Part model, mm, in its own coordinate system. A direction names the side the tool comes from. Give positions to 0.01 mm unless a question says otherwise; leave off trailing zeros. Write each loop counter-clockwise with the first axis right and the second up, starting at its lowest first coordinate (ties: lowest second). Pieces come first, ordered by that corner, then holes.
```python
from build123d import *

# Parameters (mm, degrees)
SKETCH1_R           = 1.4375
BOSS_EXTRUDE1_DEPTH = 5.999988
FILLET3_R           = 7.62
CUT_EXTRUDE2_DEPTH  = 91.763371988
FILLET5_R           = 5.5


with BuildPart() as part:
    # Sketch1 → Boss-Extrude1 (new body)
    # profile 1 of 2: a face of its own
    with BuildSketch(Plane.XY):
        with BuildLine():
            Line((-12.524548321, 23.175850862), (-8.858779162, 0))
            Line((-8.858779162, 0), (79.974319043, 0))
            Line((79.974319043, 0), (82.794220418, 17.828076701))
            ThreePointArc((82.794220418, 17.828076701), (80.81199482, 25.527902595), (73.838835056, 29.347795267))
            Line((73.838835056, 29.347795267), (-2.145190776, 36.382122067))
            ThreePointArc((-2.145190776, 36.382122067), (4.322784828, 33.16197662), (6.932987084, 26.424700516))
            ThreePointArc((6.932987084, 26.424700516), (6.181465859, 22.621328283), (4.039859015, 19.389619041))
            ThreePointArc((4.039859015, 19.389619041), (3.875471285, 19.227345924), (3.707379331, 19.06891302))
            ThreePointArc((3.707379331, 19.06891302), (-5.519878365, 16.730194284), (-12.524548321, 23.175850862))
        make_face()
        with Locations((72.917012916, 19.390373716)):
            Circle(SKETCH1_R, mode=Mode.SUBTRACT)
    # profile 2 of 2: a face of its own
    with BuildSketch(Plane.XY):
        with BuildLine():
            ThreePointArc((-2.145190776, 36.382122067), (-10.929328098, 32.604020866), (-12.524548321, 23.175850862))
            ThreePointArc((-12.524548321, 23.175850862), (-5.519878365, 16.730194284), (3.707379331, 19.06891302))
            ThreePointArc((3.707379331, 19.06891302), (3.875471285, 19.227345924), (4.039859015, 19.389619041))
            ThreePointArc((4.039859015, 19.389619041), (6.181465859, 22.621328283), (6.932987084, 26.424700516))
            ThreePointArc((6.932987084, 26.424700516), (4.322784828, 33.16197662), (-2.145190776, 36.382122067))
        make_face()
        with Locations((-3.067012916, 26.424700516)):
            Circle(SKETCH1_R, mode=Mode.SUBTRACT)
    extrude(amount=BOSS_EXTRUDE1_DEPTH)

    # Fillet3
    fillet3_edges = [part.edges().sort_by_distance(p)[0] for p in [
        (79.974319043, 0, 2.999994),
        (-8.858779162, 0, 2.999994),
    ]]
    fillet(fillet3_edges, radius=FILLET3_R)

    # Sketch3 → Cut-Extrude2 (cut, through all)
    with BuildSketch(Plane.XY.offset(5.999988)):
        Polygon((5.750849923, 35.651135125), (8.226420239, 20), (62.889119642, 20), (64.504363049, 30.211946987), align=None)
    extrude(amount=-CUT_EXTRUDE2_DEPTH, mode=Mode.SUBTRACT)

    # Fillet5
    fillet5_edges = [part.edges().sort_by_distance(p)[0] for p in [
        (5.750849923, 35.651135125, 2.999994),
        (64.504363049, 30.211946987, 2.999994),
        (62.889119642, 20, 2.999994),
        (8.226420239, 20, 2.999994),
    ]]
    fillet(fillet5_edges, radius=FILLET5_R)


solid = part.part
```
1) 3-axis set-ups, long thin cutter, end or side, ignore diameter. For faces 5 (the face through (6.95, 28.08, 3.04)), 6 (the face through (34, 14, 0)): which of +Z, -Z, +X, -X, +Y, -Y reach the whole face in a straight line?
Answers follow:
face 5: +Z, -Z, +Y
face 6: -Z, +X, -X, +Y, -Y
2) Wall check: L1, parallel to Y at x = 22, z = 0.3; L2, parallel to X at y = 27, z = 1.9; L3, parallel to X at y = 19.5, z = 2.55. Give the ranges that are in metal, low to high.
Answers follow:
L1: y = 0 to 20
L2: x = -13.05 to -4.38, -1.75 to 7.12, 64.36 to 79.4
L3: x = -11.94 to 71.48, 74.35 to 82.92
3) Saw through at B-B, the plane x = 26.5. Write the cut outline in (y, z).
Answers follow:
outline: (0, 0) - (20, 0) - (20, 6) - (0, 6) - close
4) Saw through at A-A, the plane z = 4.8. Write the cut outline in (x, y) (1 decimal), then the cut area to 3 significant figures.
Answers follow:
outline: (-12.5, 23.2) - (-9.9, 6.4) arc R7.6 ccw to (-2.3, 0) - (73.5, 0) arc R7.6 ccw to (81, 6.4) - (82.8, 17.8) arc R10 ccw to (73.8, 29.3) - (69.6, 29.7) arc R5.5 ccw to (63.7, 25.1) - (63.6, 24.6) arc R5.5 cw to (58.2, 20) - (12.9, 20) arc R5.5 cw to (7.5, 24.6) - (6.4, 31.4) arc R5.5 ccw to (1.5, 36) - (-2.1, 36.4) arc R10 ccw to start; hole circle Ø2.9 at (-3.1, 26.4); hole circle Ø2.9 at (72.9, 19.4)
area: 2,270 mm2
5) Two-plate mould, pull along Y, no slides. Class faces 1 (the face through (35, 0, 3)), 2 (the face through (-3.38, 25.02, 2.96)), 3 (the face through (73.69, 20.6, 2.96)), 4 (the face through (71.77, 29.54, 2.96)): +Y half, -Y half, draft (parallel to the pull), parting line (faces both ways), or undercut.
Answers follow:
face 1: -Y half
face 2: undercut
face 3: undercut
face 4: +Y half
6) Pin check, flat tips, straight feed: pin 1 Ø4.5 at (x, y) = (72.92, 19.39) entering from -Z; pin 2 Ø2 at (y, z) = (7.5, 4) entering from -X. Stop position of each tip, or through.
Answers follow:
pin 1: stops at z = 0
pin 2: stops at x = -10.2
7) Saw through at C-C, the plane y = 12. Write the cut outline in (x, z).
Answers follow:
outline: (-10.76, 0) - (81.87, 0) - (81.87, 6) - (-10.76, 6) - close
